Read the model definition and answer for the solid it produces. Units are mm, in the model's axes. A direction names the side the tool comes from. Give positions to 0.01 mm unless a question says otherwise; leave off trailing zeros. Order: outer loops, then holes, each group sorted by start corner. A loop starts at its lowest first (then second) coordinate and runs counter-clockwise, first axis right, second up. Notation, with made-up numbers: (25, 30) - (36, 30) arc R22 cw to (36, 69) - close; hole circle Ø2 at (72, 21.25). An arc over 180 degrees is marked (long way). Write item = value, one per line.
```python
from build123d import *

# Parameters (mm, degrees)
CROQUIS1_R                   = 12.5
SALIENTE_EXTRUIR1_DEPTH      = 3
TALADRO_DE_MARGEN_PARA_M42_D = 4.5
KEYWAY_DEPTH                 = 4


with BuildPart() as part:
    # Croquis1 → Saliente-Extruir1 (new body)
    with BuildSketch(Plane.XY):
        with BuildLine():
            Line((70, 25), (0, 25))
            ThreePointArc((0, 25), (-25, 0), (0, -25))
            Line((0, -25), (70, -25))
            ThreePointArc((70, -25), (95, 0), (70, 25))
        make_face()
        with Locations((70, 0)):
            Circle(CROQUIS1_R, mode=Mode.SUBTRACT)
    extrude(amount=SALIENTE_EXTRUIR1_DEPTH)

    # Taladro de margen para M42 (through all)
    with Locations(Plane.XY.offset(3)):
        with Locations((-21, 0), (91, 0), (-10.5, 18.186533479), (10.5, 18.186533479), (21, 0), (10.5, -18.186533479), (-10.5, -18.186533479), (80.5, -18.186533479), (59.5, -18.186533479), (49, 0), (59.5, 18.186533479), (80.5, 18.186533479)):
            Hole(TALADRO_DE_MARGEN_PARA_M42_D / 2)

    # KeySketch → Keyway (cut, through all)
    with BuildSketch(Plane(origin=(0.837491084, -0.474467987, 3), x_dir=(1, 0, 0), z_dir=(0, 0, 1))):
        with BuildLine():
            Line((-4.837491084, 12.843784864), (-4.837491084, 16.774467987))
            Line((-4.837491084, 16.774467987), (3.162508916, 16.774467987))
            Line((3.162508916, 16.774467987), (3.162508916, 12.843784864))
            ThreePointArc((3.162508916, 12.843784864), (-0.837491084, -12.525532013), (-4.837491084, 12.843784864))
        make_face()
    extrude(amount=-KEYWAY_DEPTH, mode=Mode.SUBTRACT)


solid = part.part
```
1. Determine the mould class of faces 3 (the face through (35, 25, 1)), 4 (the face through (10.988, -20.383, 1.479)), 5 (the face through (-4, 14, 2)), 6 (the face through (-24.994, 0.55, 1.479)) for opening direction Y: +Y half, -Y half, draft (parallel to the pull), parting line (faces both ways), or undercut.
Recorded:
face_3 = +Y half
face_4 = undercut
face_5 = undercut
face_6 = parting line
2. Section D-D (x = 1.5) is taken. Determine the outline of the cut face in (y, z).
Recorded:
outline = (-25, 0) - (-12.91, 0) - (-12.91, 3) - (-25, 3) - close; (16.3, 0) - (25, 0) - (25, 3) - (16.3, 3) - close
3. Section B-B (x = 21) is taken. Determine the outline of the cut face in (y, z), and give its area (4 significant figures).
Recorded:
outline = (-25, 0) - (-2.25, 0) - (-2.25, 3) - (-25, 3) - close; (2.25, 0) - (25, 0) - (25, 3) - (2.25, 3) - close
area = 136.5 mm^2
4. Flat-ended cylindrical pins translate along their axes: pin 1 (1.5 mm diameter, centred on y = 3, z = 1.5, fed in from -X); pin 2 (2.5 mm diameter, centred on x = -21, y = 0, fed in from +Z); pin 3 (6 mm diameter, centred on x = 59.5, y = 18.19, fed in from +Z); pin 4 (1.5 mm diameter, centred on y = -6.5, z = 2.5, fed in from +X). Find the tip coordinate at first contact, or state that the pin passes through.
Recorded:
pin_1 = -24.9
pin_2 = through
pin_3 = 3
pin_4 = 94.33
5. Section A-A (y = 0) is taken. Determine the outline of the cut face in (x, z).
Recorded:
outline = (-25, 0) - (-23.25, 0) - (-23.25, 3) - (-25, 3) - close; (-18.75, 0) - (-13, 0) - (-13, 3) - (-18.75, 3) - close; (13, 0) - (18.75, 0) - (18.75, 3) - (13, 3) - close; (23.25, 0) - (46.75, 0) - (46.75, 3) - (23.25, 3) - close; (51.25, 0) - (57.5, 0) - (57.5, 3) - (51.25, 3) - close; (82.5, 0) - (88.75, 0) - (88.75, 3) - (82.5, 3) - close; (93.25, 0) - (95, 0) - (95, 3) - (93.25, 3) - close
6. Section C-C (x = 59.5) is taken. Determine the outline of the cut face in (y, z), and give its area (3 significant figures).
Recorded:
outline = (-25, 0) - (-20.44, 0) - (-20.44, 3) - (-25, 3) - close; (-15.94, 0) - (-6.78, 0) - (-6.78, 3) - (-15.94, 3) - close; (6.78, 0) - (15.94, 0) - (15.94, 3) - (6.78, 3) - close; (20.44, 0) - (25, 0) - (25, 3) - (20.44, 3) - close
area = 82.3 mm^2
7. Straight lines are drawn through the part: L1, parallel to Y at x = 70, z = 1.5; L2, parallel to Y at x = 59.5, z = 1; L3, parallel to Y at x = -10.5, z = 1.95. For each, find the intervals that lie inside material, in ascending order. Write a range as [from, to].
Recorded:
L1 = [-25, -12.5], [12.5, 25]
L2 = [-25, -20.44], [-15.94, -6.78], [6.78, 15.94], [20.44, 25]
L3 = [-22.69, -20.44], [-15.94, -7.66], [7.66, 15.94], [20.44, 22.69]
8. For faces 1 (the face through (35, -25, 1)), 2 (the face through (4, 14, 2)), determine the directions among +Z, -Z, +X, -X, +Y, -Y from which every point of the face is accessible in a straight line to the end or side of a thin tool.
Recorded:
face_1 = +Z, -Z, +X, -X, -Y
face_2 = +Z, -Z
